Model file for the job. Use its own axes, mm. Face numbers are marked on the shaded views. Round coordinates to 2 decimals unless told otherwise and drop trailing zeros. Order: outer loops, then holes, each group sorted by start corner. A loop starts at its lowest first (then second) coordinate and runs counter-clockwise, first axis right, second up. Notation, with made-up numbers: (-21.75, 26.5) - (7.25, 26.5) arc R22 cw to (7.25, 36.5) - close; hole circle Ø2 at (64.25, 44). An arc over 180 degrees is marked (long way). Answer as CSV lines item,"result". Start each with the question number.
1. Band-saw the part on D-D on x = -15. List the corners of the cut face in (y, z), then the cut area to 3 significant figures.
2. Band-saw the part on C-C on y = 1.9. List the corners of the cut face in (x, z), then the cut area to 3 significant figures.
3. Wall check: line 1 along Z through (x, y) = (-9.75, 2.3); line 2 along Z through (x, y) = (-11.25, 0.55); line 3 along X through (y, z) = (3.95, -14). Give the ranges that are in metal, low to high. Write a range as [from, to].
4. Pull direction Z, two halves, no side cores. Call the marked faces 1, 2, 3 and 4: released by +Z, released by -Z, zero draft, split by the parting line, or undercut.
5. Band-saw the part on B-B on z = -13.5. List the corners of the cut face in (x, y), then the cut area to 3 significant figures.
6. Pin check, flat tip, straight feed: pin 1 Ø1 at (y, z) = (0.5, -14) entering from -X. Stop position of the tip, or through.
7. Band-saw the part on A-A on x = -9. List the corners of the cut face in (y, z), then the cut area to 3 significant figures.
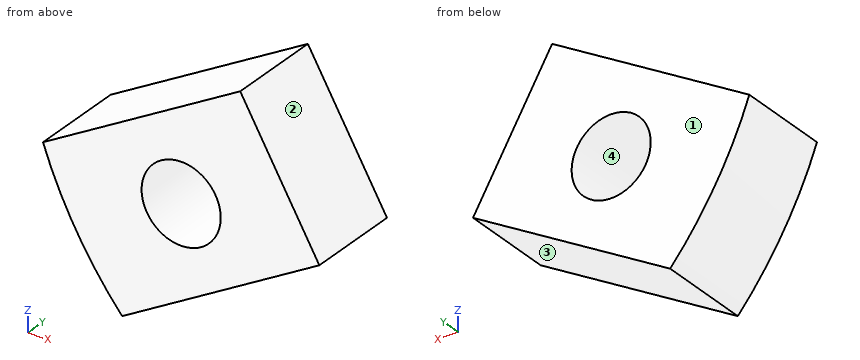
Autodesk Inventor part; units mm, degrees
ref_plane "YZ Plane" through (0, 0, 0) normal (1, 0, 0) x (0, 1, 0)
ref_plane "XZ Plane" through (0, 0, 0) normal (0, 1, 0) x (-1, 0, 0)
ref_plane "XY Plane" through (0, 0, 0) normal (0, 0, 1) x (1, 0, 0)
sketch "Sketch7" plane through (0, 0, 0) normal (0, 1, 0) x (-1, 0, 0)
  circle A0 centre (-6.4493, -2.4672) radius 27.5
  circle A1 centre (-6.4493, -2.4672) radius 3.05
  line L0 (-6.4493, -2.4672) -> (-6.4493, 25.0328)
  line L1 (-11.4493, 39.8773) -> (-1.4493, 39.8773)
  line L2 (-1.4493, 39.8773) -> (-1.4493, 10.1882)
  line L3 (-1.4493, 10.1882) -> (-11.4493, 10.1882)
  line L4 (-11.4493, 10.1882) -> (-11.4493, 39.8773)
  line L5 (-11.4493, 39.8773) -> (-1.4493, 10.1882) construction
  line L6 (-1.4493, 39.8773) -> (-11.4493, 10.1882) construction
  line L7 (-45.6207, -19.3094) -> (-19.9093, -4.4649)
  line L8 (-19.9093, -4.4649) -> (-14.9093, -13.1251)
  line L9 (-14.9093, -13.1251) -> (-40.6207, -27.9696)
  line L10 (27.7221, -27.9696) -> (2.0107, -13.1251)
  line L11 (2.0107, -13.1251) -> (7.0107, -4.4649)
  line L12 (7.0107, -4.4649) -> (32.7221, -19.3094)
  point P0 (0, 0)
  point P1 (14.4694, -20.3182)
  point P2 (19.4694, -11.6579)
  dimension "d8" = 360
extrude "Extrusion2" add sketch "Sketch7" along normal blind 6 contours A0 L10 L11 L12
sketch "Sketch8" plane through (0, 6, 0) normal (0, 1, 0) x (1, 0, 0)
  arc A0 (-14.4694, 20.3182) -> (-19.4694, 11.6579) centre (6.4493, 2.4672) ccw
  line L0 (-19.4694, 11.6579) -> (-7.0107, 4.4649)
  line L1 (-14.4694, 20.3182) -> (-19.4694, 11.6579)
  circle A1 centre (-10.7401, 12.3915) radius 2.5
  point P0 (0, 0)
  dimension "d11" = 5
extrude "Extrusion3" cut sketch "Sketch8" against normal through all contours A1
sketch "Sketch12" plane through (0, 0, 0) normal (0, -1, 0) x (1, 0, 0)
  line L0 (-2.0107, -13.1251) -> (-14.4694, -20.3182)
  line L1 (-19.4694, -11.6579) -> (-7.0107, -4.4649)
  line L2 (-14.4694, -20.3182) -> (-19.4694, -11.6579)
  point P0 (0, 0)
equation "\"BendRadius\" = Thickness"
equation "\"BendReliefWidth\" = Thickness"
equation "\"BendReliefDepth\" = 0.5 * Thickness"
equation "\"CornerReliefSize\" = 4 * Thickness"
equation "\"MinimumRemnant\" = 2 * Thickness"
equation "\"TransitionRadius\" = BendRadius"
equation "\"JacobiRadiusSize\" = BendRadius"
equation "\"GapSize\" = Thickness"
Reply:
1,outline,"(0, -19.68) - (6, -19.68) - (6, -9.08) - (0, -9.08) - close"
1,area,"63.6 mm2"
2,outline,"(-19.47, -11.66) arc R27.5 ccw to (-14.47, -20.32) - (-2.01, -13.13) - (-7.01, -4.46) - close; hole circle Ø5 at (-10.74, -12.39)"
2,area,"127 mm2"
3,line 1,"z = [-17.59, -14.69], [-10.1, -6.05]"
3,line 2,"z = [-18.46, -14.84], [-9.94, -6.91]"
3,line 3,"x = [-18.52, -12.65], [-8.83, -3.53]"
4,face 1,"zero draft"
4,face 2,"released by +Z"
4,face 3,"released by -Z"
4,face 4,"undercut"
5,outline,"(-18.74, 0) - (-12.98, 0) - (-12.98, 6) - (-18.74, 6) - close; (-8.5, 0) - (-2.66, 0) - (-2.66, 6) - (-8.5, 6) - close"
5,area,"69.6 mm2"
6,pin 1,"stops at x = -18.74"
7,outline,"(0, -17.16) - (6, -17.16) - (6, -14.19) - (0, -14.19) - close; (0, -10.6) - (6, -10.6) - (6, -5.61) - (0, -5.61) - close"
7,area,"47.7 mm2"
